```python
from build123d import *

# Parameters (mm, degrees)
CHAMFER2_SIZE = 0.25


with BuildPart() as part:
    # Sketch1 → Revolve1 (revolve)
    with BuildSketch(Plane(origin=(0, 0, 0), x_dir=(1, 0, 0), z_dir=(0, 1, 0))):
        Polygon((-4, 25), (-4, 15), (-20, 0), (-20, -8), (-18.5, -8), (-18.5, 0), (-3.25, 14.296875), (-3.25, 25), align=None)
    revolve(axis=Axis((0, 0, 0), (0, 0, -1)))

    # Chamfer2
    chamfer2_edges = [part.edges().sort_by_distance(p)[0] for p in [
        (4, 0, -25),
    ]]
    chamfer(chamfer2_edges, length=CHAMFER2_SIZE)


solid = part.part
```
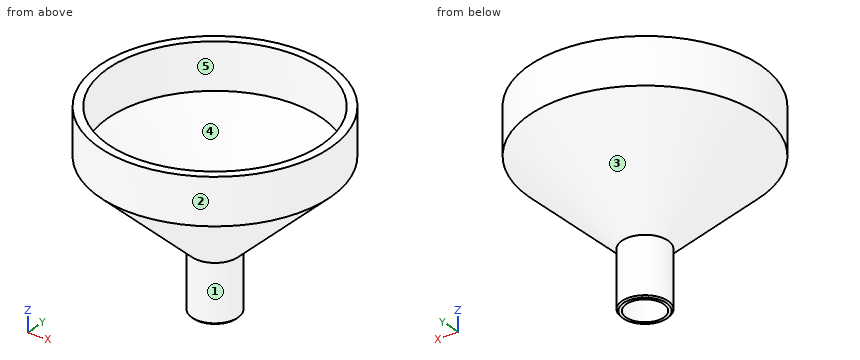
For this review, take the finished solid that the model builds, in its own axes (mm). Face numbers are marked on the shaded views. A direction names the side the tool comes from. Round coordinates to 2 decimals unless told otherwise and drop trailing zeros. Write each loop counter-clockwise with the first axis right and the second up, starting at its lowest first coordinate (ties: lowest second). Pieces come first, ordered by that corner, then holes. Notation, with made-up numbers: (-27, -29.5) -> (-21, -29.5) arc R21 ccw to (-21, -10.5) -> close; hole circle Ø2 at (-40, -6). An arc over 180 degrees is marked (long way). Use one line per item in the form item = value.
1) To check wall thickness, follow L1, parallel to Y at x = 0, z = 5.75; L2, parallel to Y at x = 0, z = -17; L3, parallel to X at y = -7, z = -9.5. State the ranges of each line that lie inside material, in increasing order. Write a range as from..to.
Found:
L1 = -20..-18.5, 18.5..20
L2 = -4..-3.25, 3.25..4
L3 = -6.95..-4.58, 4.58..6.95
2) Take a section at D-D, the plane z = 2. Write out the cut boundary in (x, y), and give its area (3 significant figures).
Found:
outline = circle Ø40 at (0, 0); hole circle Ø37 at (0, 0)
area = 181 mm2
3) Tool access review of the marked faces 1 and 2: name each direction out of +Z, -Z, +X, -X, +Y, -Y from which nothing blocks a thin tool from reaching the whole face with its end or side.
Found:
face_1 = -Z
face_2 = +Z, -Z
4) Mouldability with a two-part tool opening along X and no side actions: class the marked faces 3, 4 and 5 as +X half, -X half, draft (parallel to the pull), parting line (faces both ways), or undercut.
Found:
face_3 = parting line
face_4 = undercut
face_5 = undercut
5) Take a section at A-A, the plane y = 0. Write out the cut boundary in (x, z).
Found:
outline = (-20, 0) -> (-4, -15) -> (-4, -24.75) -> (-3.75, -25) -> (-3.25, -25) -> (-3.25, -14.3) -> (-18.5, 0) -> (-18.5, 8) -> (-20, 8) -> close; (3.25, -25) -> (3.75, -25) -> (4, -24.75) -> (4, -15) -> (20, 0) -> (20, 8) -> (18.5, 8) -> (18.5, 0) -> (3.25, -14.3) -> close
6) Take a section at C-C, the plane z = -17.5. Write out the cut boundary in (x, y).
Found:
outline = circle Ø8 at (0, 0); hole circle Ø6.5 at (0, 0)
7) Clearance check with flat-ended pins moving along their axes: pin 1 (4 mm diameter, centred on y = -6.5, z = -4.5, fed in from +X); pin 2 (2 mm diameter, centred on y = 0, z = -4, fed in from +X); pin 3 (2 mm diameter, centred on x = -3.5, y = 11, fed in from -Z). State where each tip first meets the part, or that it passes through.
Found:
pin_1 = 16.19
pin_2 = 16.8
pin_3 = -8.87
